For this review, take the finished solid that the model builds, in its own axes (mm). A direction names the side the tool comes from. Give positions to 0.01 mm unless a question says otherwise; leave off trailing zeros. Loops run counter-clockwise (first coordinate to the right, second up) from the corner with the lowest first, then second, coordinate; pieces in that order, holes last. Notation, with made-up numbers: (-35.75, 9) - (23.25, 9) arc R18 ccw to (23.25, 37) - close; hole circle Ø6 at (2, -22.75). An arc over 180 degrees is marked (long way). Answer as CSV lines item,"result".
Autodesk Inventor part; units mm, degrees
ref_plane "YZ Plane" through (0, 0, 0) normal (1, 0, 0) x (0, 1, 0)
ref_plane "XZ Plane" through (0, 0, 0) normal (0, 1, 0) x (-1, 0, 0)
ref_plane "XY Plane" through (0, 0, 0) normal (0, 0, 1) x (1, 0, 0)
sketch "Sketch1" plane through (0, 0, 0) normal (0, 0, 1) x (1, 0, 0)
  line L0 (0, 244.475) -> (19.05, 244.475)
  line L1 (19.05, 244.475) -> (19.05, 225.425)
  line L2 (19.05, 225.425) -> (0, 225.425)
  line L3 (0, 225.425) -> (0, 244.475)
  line L4 (19.05, 168.275) -> (0, 168.275)
  line L5 (0, 168.275) -> (0, 149.225)
  line L6 (0, 149.225) -> (19.05, 149.225)
  line L7 (19.05, 149.225) -> (19.05, 168.275)
  line L8 (0, 130.175) -> (19.05, 130.175)
  line L9 (19.05, 130.175) -> (19.05, 111.125)
  line L10 (19.05, 111.125) -> (0, 111.125)
  line L11 (0, 111.125) -> (0, 130.175)
  line L12 (0, 206.375) -> (19.05, 206.375)
  line L13 (19.05, 206.375) -> (19.05, 187.325)
  line L14 (19.05, 187.325) -> (0, 187.325)
  line L15 (0, 187.325) -> (0, 206.375)
  line L16 (0, 92.075) -> (19.05, 92.075)
  line L17 (19.05, 92.075) -> (19.05, 73.025)
  line L18 (19.05, 73.025) -> (0, 73.025)
  line L19 (0, 73.025) -> (0, 92.075)
  line L20 (0, 53.975) -> (19.05, 53.975)
  line L21 (19.05, 53.975) -> (19.05, 34.925)
  line L22 (19.05, 34.925) -> (0, 34.925)
  line L23 (0, 34.925) -> (0, 53.975)
  line L24 (0, 15.875) -> (19.05, 15.875)
  line L25 (19.05, 15.875) -> (19.05, -3.175)
  line L26 (19.05, -3.175) -> (0, -3.175)
  line L27 (0, -3.175) -> (0, 15.875)
  line L28 (0, 244.475) -> (206.375, 244.475)
  line L29 (206.375, 244.475) -> (206.375, 0)
  line L30 (206.375, 0) -> (0, 0)
  line L31 (19.05, 244.475) -> (19.05, 0)
  line L32 (206.375, 244.475) -> (19.05, 244.475)
  line L33 (19.05, 244.475) -> (19.05, 0)
  line L34 (19.05, 0) -> (206.375, 0)
  line L35 (206.375, 0) -> (206.375, 244.475)
  dimension "d0" = 19.05
  dimension "d1" = 19.05
  dimension "d3" = 19.05
  dimension "d4" = 19.05
  dimension "d5" = 19.05
  dimension "d6" = 19.05
  dimension "d7" = 19.05
  dimension "d8" = 19.05
  dimension "d9" = 19.05
  dimension "d10" = 19.05
  dimension "d11" = 19.05
  dimension "d12" = 19.05
  dimension "d13" = 19.05
  dimension "d14" = 19.05
  dimension "d15" = 19.05
  dimension "d16" = 19.05
  dimension "d17" = 19.05
  dimension "d18" = 19.05
  dimension "d19" = 19.05
  dimension "d21" = 206.375
  dimension "d22" = 244.475
  dimension "d23" = 206.375
extrude "Extrusion1" add sketch "Sketch1" along normal blind 19.05 contours L0 L1 L2 L3 | L28 L29 L30 L25 L31 L21 L17 L9 L7 L13 L1 | L13 L14 L15 L12 | L30 L27 L24 L25 | L7 L6 L5 L4 | L22 L23 L20 L21 | L9 L10 L11 L8 | L18 L19 L16 L17
mirror "Mirror1" about plane through (206.375, 0, 0) normal (1, 0, 0) of "Extrusion1"
sketch "Sketch2" plane through (0, 0, 19.05) normal (0, 0, 1) x (1, 0, 0)
  line L0 (412.75, 244.475) -> (412.75, 225.425)
  line L1 (0, 244.475) -> (412.75, 244.475)
  line L2 (0, 244.475) -> (0, 225.425)
  line L3 (19.05, 244.475) -> (393.7, 244.475)
  line L4 (393.7, 244.475) -> (393.7, 228.6)
  line L5 (393.7, 228.6) -> (19.05, 228.6)
  line L6 (19.05, 228.6) -> (19.05, 244.475)
  dimension "d26" = 19.05
  dimension "d27" = 19.05
  dimension "d28" = 15.875
extrude "Extrusion2" cut sketch "Sketch2" against normal blind 9.525
properties part number "deep_end" material "Wood (Birch)"
1) Draft analysis for pull direction X (two halves, no side actions). For faces 6 (the flat face through (19.05, 140, 9)), 7 (the flat face through (204, 237, 9.525)), 8 (the flat face through (393.7, 101, 9)), state which applies: pulls with the +X half, pulls with the -X half, needs draft (parallel to the pull), parting line crosses it, or undercut.
From the geometry:
face 6,"pulls with the -X half"
face 7,"undercut"
face 8,"pulls with the +X half"
2) Machinability: for faces 1 (the flat face through (412.75, 83, 9)), 2 (the flat face through (9, 130.175, 9)), 3 (the flat face through (393.7, 237, 14)), 4 (the flat face through (0, 44, 9)), 5 (the flat face through (393.7, 140, 9)), which of the approach directions +Z, -Z, +X, -X, +Y, -Y give a long, thin tool a straight path to every point of the face, cutting with its end or side? Answer none if there is none.
From the geometry:
face 1,"+Z, -Z, +X, +Y, -Y"
face 2,"+Z, -Z, -X"
face 3,"+Z, +Y"
face 4,"+Z, -Z, -X, +Y, -Y"
face 5,"+Z, -Z, +X"
3) Insertion check: P1, Ø9.5, axis at y = 177.5, z = 11, coming from the -X side; P2, Ø8, axis at x = 233.5, y = 237.5, coming from the +Z side (3 decimals); P3, Ø3, axis at y = 56, z = 11.5, coming from the +X side. Each pin has a flat end and moves straight along its axis. Give the tip position at first contact, or say it passes through.
From the geometry:
P1,"stops at x = 19.05"
P2,"stops at z = 9.525"
P3,"stops at x = 393.7"
4) Consider section B-B on y = 220. Write out the cut boundary in (x, z).
From the geometry:
outline,"(19.05, 0) - (393.7, 0) - (393.7, 19.05) - (19.05, 19.05) - close"
5) Wall thickness on line 1 (X direction, y = 144.5, z = 8.25); line 2 (Y direction, x = 326.5, z = 11.25): over which ranges is each line inside the solid? List them lowest first. Write a range as from..to.
From the geometry:
line 1,"x = 19.05..393.7"
line 2,"y = 0..228.6"
6) Consider section A-A on x = 211. Write out the cut boundary in (y, z) (3 decimals).
From the geometry:
outline,"(0, 0) - (244.475, 0) - (244.475, 9.525) - (228.6, 9.525) - (228.6, 19.05) - (0, 19.05) - close"
